The listing builds one solid part. Answer for the finished solid, in the listing's coordinates (mm). Face numbers are marked on the shaded views. A direction names the side the tool comes from. Round coordinates to 2 decimals unless told otherwise and drop trailing zeros. Loops run counter-clockwise (first coordinate to the right, second up) from the corner with the lowest first, then second, coordinate; pieces in that order, holes last. Notation, with made-up numbers: (84.25, -19.5) -> (126.25, -19.5) arc R19 ccw to (126.25, -2.5) -> close; hole circle Ø6 at (69.5, 23.5). An arc over 180 degrees is marked (long way). Use a Markdown table: item, result. Add a question column.
Q1. Section A-A on z = 0 is taken. Give the vertices of the cut face in (x, y), then the cut area to 3 significant figures.
Q2. Which of the six approach directions +Z, -Z, +X, -X, +Y, -Y give full straight-line access (tool end or side, diameter ignored) to the marked faces 4, 5 and 6?
Q3. Section D-D on x = -1 is taken. Give the vertices of the cut face in (y, z), then the cut area to 3 significant figures.
Q4. Consider line 1 (Z direction, x = -28.95, y = 6); line 2 (X direction, y = 7, z = 2); line 3 (X direction, y = 2.5, z = -6). Determine where each line is inside the solid, lowest interval first.
Q5. Given pin 1 Ø5 at (y, z) = (7.5, 6.5) entering from +X; pin 2 Ø2 at (x, z) = (-21.5, -13.5) entering from +Y; pin 3 Ø4.5 at (x, z) = (-28.95, -23) entering from -Y, each flat-ended and moving along its own axis, determine where each tip first touches the part or whether it passes through.
Q6. Section B-B on y = 6.75 is taken. Give the number of separate pieces and of enclosed holes in the cut face, then the cut area to 3 significant figures.
Q7. For a pull along Z with two mould halves and no side action, classify the marked faces 1, 2 and 3 as released by +Z, released by -Z, zero draft, split by the parting line, or undercut.
from build123d import *

# Parameters (mm, degrees)
SKETCH1_W           = 48.9
SKETCH1_H           = 55
SKETCH1_W_2         = 45.9
SKETCH1_H_2         = 9.4
SKETCH1_H_3         = 33.2
BOSS_EXTRUDE1_DEPTH = 4
SKETCH2_W           = 1.5
SKETCH2_H           = 33.2
SKETCH2_W_2         = 5
SKETCH2_H_2         = 1.5
SKETCH2_H_3         = 9.4
SKETCH2_W_3         = 2.2
BOSS_EXTRUDE2_DEPTH = 6
SKETCH4_R           = 4.5
SKETCH4_R_2         = 1.75
BOSS_EXTRUDE3_DEPTH = 10
FILLET1_R           = 1
CUT_EXTRUDE1_DEPTH  = 2.75


with BuildPart() as part:
    # Sketch1 → Boss-Extrude1 (new body)
    with BuildSketch(Plane(origin=(0, 0, 0), x_dir=(1, 0, 0), z_dir=(0, 1, 0))):
        Rectangle(SKETCH1_W, SKETCH1_H)
        Polygon((22.95, 26), (22.95, 16.6), (22.95, -16.6), (22.95, -26), (-22.95, -26), (-22.95, -16.6), (-22.95, 16.6), (-22.95, 26), align=None, mode=Mode.SUBTRACT)
        with Locations((0, 21.3)):
            Rectangle(SKETCH1_W_2, SKETCH1_H_2)
        Rectangle(SKETCH1_W_2, SKETCH1_H_3)
        with Locations((0, -21.3)):
            Rectangle(SKETCH1_W_2, SKETCH1_H_2)
    extrude(amount=BOSS_EXTRUDE1_DEPTH)

    # Sketch2 → Boss-Extrude2 (add)
    with BuildSketch(Plane(origin=(0, 4, 0), x_dir=(1, 0, 0), z_dir=(0, 1, 0))):
        Polygon((-24.45, 16.6), (-22.95, 16.6), (-22.95, 26), (-20.75, 26), (-20.75, 27.5), (-24.45, 27.5), align=None)
        with Locations((-23.7, 0)):
            Rectangle(SKETCH2_W, SKETCH2_H)
        Polygon((-22.95, -26), (-22.95, -16.6), (-24.45, -16.6), (-24.45, -27.5), (-20.75, -27.5), (-20.75, -26), align=None)
        with Locations((-7.75, -26.75)):
            Rectangle(SKETCH2_W_2, SKETCH2_H_2)
        with Locations((7.75, -26.75)):
            Rectangle(SKETCH2_W_2, SKETCH2_H_2)
        Polygon((24.45, -16.6), (22.95, -16.6), (22.95, -26), (20.75, -26), (20.75, -27.5), (24.45, -27.5), align=None)
        with Locations((23.7, 0)):
            Rectangle(SKETCH2_W, SKETCH2_H)
        Polygon((22.95, 26), (22.95, 16.6), (24.45, 16.6), (24.45, 27.5), (20.75, 27.5), (20.75, 26), align=None)
        with Locations((7.75, 26.75)):
            Rectangle(SKETCH2_W_2, SKETCH2_H_2)
        with Locations((-7.75, 26.75)):
            Rectangle(SKETCH2_W_2, SKETCH2_H_2)
        with Locations((-7.75, 21.3)):
            Rectangle(SKETCH2_W_2, SKETCH2_H_3)
        with Locations((7.75, 21.3)):
            Rectangle(SKETCH2_W_2, SKETCH2_H_3)
        with Locations((7.75, -21.3)):
            Rectangle(SKETCH2_W_2, SKETCH2_H_3)
        with Locations((-7.75, -21.3)):
            Rectangle(SKETCH2_W_2, SKETCH2_H_3)
        with Locations((-21.85, 21.3)):
            Rectangle(SKETCH2_W_3, SKETCH2_H_3)
        with Locations((21.85, 21.3)):
            Rectangle(SKETCH2_W_3, SKETCH2_H_3)
        with Locations((21.85, -21.3)):
            Rectangle(SKETCH2_W_3, SKETCH2_H_3)
        with Locations((-21.85, -21.3)):
            Rectangle(SKETCH2_W_3, SKETCH2_H_3)
    extrude(amount=BOSS_EXTRUDE2_DEPTH)

    # Sketch4 → Boss-Extrude3 (add)
    with BuildSketch(Plane.XZ):
        with BuildLine():
            Line((-24.45, 27.5), (-28.95, 27.5))
            ThreePointArc((-28.95, 27.5), (-25.768019485, 26.181980515), (-24.45, 23))
            Line((-24.45, 23), (-24.45, 27.5))
        make_face()
        with BuildLine():
            Line((-24.45, 18.5), (-24.45, 23))
            ThreePointArc((-24.45, 23), (-25.768019485, 19.818019485), (-28.95, 18.5))
            Line((-28.95, 18.5), (-24.45, 18.5))
        make_face()
        with Locations((-28.95, 23)):
            Circle(SKETCH4_R)
        with Locations((-28.95, 23)):
            Circle(SKETCH4_R_2, mode=Mode.SUBTRACT)
        with BuildLine():
            ThreePointArc((24.45, 22.999999999), (25.768019484, 26.181980515), (28.95, 27.5))
            Line((28.95, 27.5), (24.45, 27.5))
            Line((24.45, 27.5), (24.45, 22.999999999))
        make_face()
        with Locations((28.95, 23)):
            Circle(SKETCH4_R)
        with Locations((28.95, 23)):
            Circle(SKETCH4_R_2, mode=Mode.SUBTRACT)
        with BuildLine():
            ThreePointArc((28.95, 18.5), (25.768019485, 19.818019484), (24.45, 22.999999999))
            Line((24.45, 22.999999999), (24.45, 18.5))
            Line((24.45, 18.5), (28.95, 18.5))
        make_face()
        with Locations((28.95, -23)):
            Circle(SKETCH4_R)
        with Locations((28.95, -23)):
            Circle(SKETCH4_R_2, mode=Mode.SUBTRACT)
        with BuildLine():
            ThreePointArc((28.95, -27.5), (25.768019485, -26.181980515), (24.45, -23))
            Line((24.45, -23), (24.45, -27.5))
            Line((24.45, -27.5), (28.95, -27.5))
        make_face()
        with BuildLine():
            Line((28.95, -18.5), (24.45, -18.5))
            Line((24.45, -18.5), (24.45, -23))
            ThreePointArc((24.45, -23), (25.768019485, -19.818019485), (28.95, -18.5))
        make_face()
        with BuildLine():
            Line((-24.45, -27.5), (-24.45, -23))
            ThreePointArc((-24.45, -23), (-25.768019485, -26.181980515), (-28.95, -27.5))
            Line((-28.95, -27.5), (-24.45, -27.5))
        make_face()
        with BuildLine():
            Line((-24.45, -23), (-24.45, -18.5))
            Line((-24.45, -18.5), (-28.95, -18.5))
            ThreePointArc((-28.95, -18.5), (-25.768019485, -19.818019485), (-24.45, -23))
        make_face()
        with Locations((-28.95, -23)):
            Circle(SKETCH4_R)
        with Locations((-28.95, -23)):
            Circle(SKETCH4_R_2, mode=Mode.SUBTRACT)
    extrude(amount=-BOSS_EXTRUDE3_DEPTH)

    # Fillet1
    fillet1_edges = [part.edges().sort_by_distance(p)[0] for p in [
        (-5.25, 4, -22.05),
        (10.25, 4, -22.05),
        (10.25, 4, 22.05),
        (-5.25, 4, 22.05),
        (-20.75, 4, -22.05),
        (-20.75, 4, 22.05),
    ]]
    fillet(fillet1_edges, radius=FILLET1_R)

    # Sketch5 → Cut-Extrude1 (cut)
    with BuildSketch(Plane.XZ):
        Polygon((-28.95, 19.709103466), (-26.1, 21.354551733), (-26.1, 24.645448267), (-28.95, 26.290896534), (-31.8, 24.645448267), (-31.8, 21.354551733), align=None)
        Polygon((31.8, 21.354551733), (28.95, 19.709103466), (26.1, 21.354551733), (26.1, 24.645448267), (28.95, 26.290896534), (31.8, 24.645448267), align=None)
        Polygon((31.8, -21.354551733), (28.95, -19.709103466), (26.1, -21.354551733), (26.1, -24.645448267), (28.95, -26.290896534), (31.8, -24.645448267), align=None)
        Polygon((-31.8, -21.354551733), (-28.95, -19.709103466), (-26.1, -21.354551733), (-26.1, -24.645448267), (-28.95, -26.290896534), (-31.8, -24.645448267), align=None)
    extrude(amount=-CUT_EXTRUDE1_DEPTH, mode=Mode.SUBTRACT)


solid = part.part
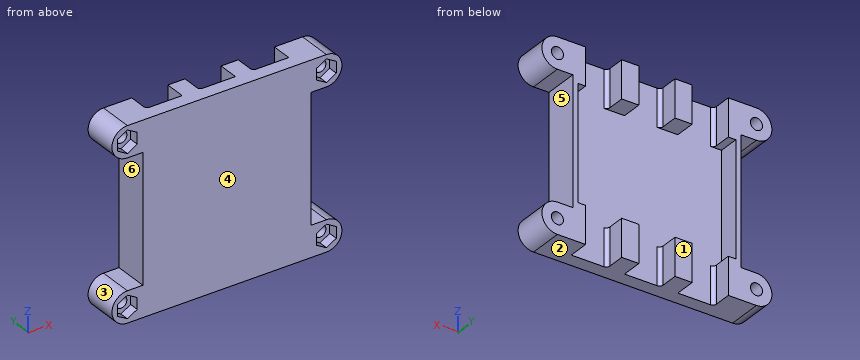
Checked values:
| question | item | result |
|---|---|---|
| 1 | outline | (-24.45, 0) -> (24.45, 0) -> (24.45, 10) -> (22.95, 10) -> (22.95, 4) -> (-22.95, 4) -> (-22.95, 10) -> (-24.45, 10) -> close |
| 1 | area | 214 mm2 |
| 2 | face 4 | +Z, -Z, +X, -X, -Y |
| 2 | face 5 | +X, +Y, -Y |
| 2 | face 6 | -X, +Y, -Y |
| 3 | outline | (0, -27.5) -> (4, -27.5) -> (4, 27.5) -> (0, 27.5) -> close |
| 3 | area | 220 mm2 |
| 4 | line 1 | z = -27.5 to -24.75, -21.25 to -18.5, 18.5 to 21.25, 24.75 to 27.5 |
| 4 | line 2 | x = -24.45 to -22.95, 22.95 to 24.45 |
| 4 | line 3 | x = -24.45 to 24.45 |
| 5 | pin 1 | stops at x = 24.45 |
| 5 | pin 2 | stops at y = 4 |
| 5 | pin 3 | stops at y = 2.75 |
| 6 | separate pieces | 6 |
| 6 | enclosed holes | 4 |
| 6 | area | 730 mm2 |
| 7 | face 1 | zero draft |
| 7 | face 2 | released by -Z |
| 7 | face 3 | undercut |
